Verification items for the finished model (mm, model axes). Face numbers are marked on the shaded views. Give positions to 0.01 mm unless a question says otherwise; leave off trailing zeros. Write each loop counter-clockwise with the first axis right and the second up, starting at its lowest first coordinate (ties: lowest second). Pieces come first, ordered by that corner, then holes. Notation, with made-up numbers: (29, 34.5) -> (77, 34.5) arc R17 ccw to (77, 53.5) -> close; hole circle Ø8 at (23, 55.25). An arc over 180 degrees is marked (long way). Use one line per item in the form item = value. Start each with the question number.
(1) Release check for a two-part mould opening along X. For the marked faces 1, 2 and 3 record: pulls with the +X half, pulls with the -X half, needs draft (parallel to the pull), parting line crosses it, or undercut.
(2) Scan lines: L1, parallel to Z at x = 52.5, y = 22; L2, parallel to X at y = 8.5, z = -28.25; L3, parallel to Y at x = 57, z = -19. Record each from-to range of solid material in increasing order.
(3) Section check B-B, the plane y = 15.5. Record the cut outline in (x, z).
(4) Depth check by flat-ended pin: pin 1 Ø4 at (y, z) = (20, -25) entering from -X; pin 2 Ø8 at (y, z) = (15.5, -28) entering from +X; pin 3 Ø2 at (x, z) = (41.5, -21) entering from +Y. Enter the tip coordinate at first touch or a pass-through.
(5) Section check A-A, the plane y = 2. Record the cut outline in (x, z).
from build123d import *

# Parameters (mm, degrees)
BOSS_EXTRUDE1_DEPTH             = 26
CUT_EXTRUDE1_DEPTH              = 26
CUT_EXTRUDE2_DEPTH              = 26
FILLET1_R                       = 5
M5_TAPPED_HOLE1_D               = 4.2
M5_TAPPED_HOLE1_DEPTH           = 6
M5_TAPPED_HOLE1_TIP             = 1.2618073
M5_TAPPED_HOLE1_ON_FACE_2_D     = 4.2
M5_TAPPED_HOLE1_ON_FACE_2_DEPTH = 6
M5_TAPPED_HOLE1_ON_FACE_2_TIP   = 1.2618073


with BuildPart() as part:
    # 草图1 → Boss-Extrude1 (new body)
    with BuildSketch(Plane(origin=(0, 0, 0), x_dir=(1, 0, 0), z_dir=(0, 1, 0))):
        Polygon((35.23935759, 18.286975519), (57.88435759, 18.286975519), (54.914973752, 35.127188096), (32.269973752, 35.127188096), align=None)
        Polygon((35.23935759, 18.286975519), (35.922187891, 14.414452446), (57.88435759, 18.286975519), align=None)
    extrude(amount=BOSS_EXTRUDE1_DEPTH)

    # Sketch1 → Cut-Extrude1 (cut)
    with BuildSketch(Plane(origin=(-1.381830042, 0, -7.836747596), x_dir=(0.984807753012208, 0, -0.17364817766693116), z_dir=(0.17364817766693116, 0, 0.984807753012208))):
        with BuildLine():
            Line((39.529978324, 0), (58.529978324, 0))
            ThreePointArc((58.529978324, 0), (49.029978324, 9.5), (39.529978324, 0))
        make_face()
    extrude(amount=-CUT_EXTRUDE1_DEPTH, mode=Mode.SUBTRACT)

    # Sketch2 → Cut-Extrude2 (cut)
    with BuildSketch(Plane(origin=(0, 26, 0), x_dir=(1, 0, 0), z_dir=(0, 1, 0))):
        Polygon((35.23935759, 18.286975519), (35.922187891, 14.414452446), (57.88435759, 18.286975519), align=None)
    extrude(amount=-CUT_EXTRUDE2_DEPTH, mode=Mode.SUBTRACT)

    # Fillet1
    fillet1_edges = [part.edges().sort_by_distance(p)[0] for p in [
        (43.592473752, 26, -35.127188096),
        (46.56185759, 26, -18.286975519),
    ]]
    fillet(fillet1_edges, radius=FILLET1_R)

    # M5 Tapped Hole1
    with Locations(Plane(origin=(33.670475294, 21, -27.184549163), x_dir=(-0.173648177667, 0, -0.984807753012), z_dir=(-0.984807753012, 0, 0.173648177667))):
        with Locations((0, 0)):
            Hole(M5_TAPPED_HOLE1_D / 2, depth=M5_TAPPED_HOLE1_DEPTH)
            with Locations((0, 0, -(M5_TAPPED_HOLE1_DEPTH + M5_TAPPED_HOLE1_TIP / 2))):  # 118° drill point
                Cone(0, M5_TAPPED_HOLE1_D / 2, M5_TAPPED_HOLE1_TIP, mode=Mode.SUBTRACT)

    # M5 Tapped Hole1 on face 2
    with Locations(Plane(origin=(56.507099646, 21, -26.097793462), x_dir=(0.17364796312, 0, 0.984807790843), z_dir=(0.984807790843, 0, -0.17364796312))):
        with Locations((0, 0)):
            Hole(M5_TAPPED_HOLE1_ON_FACE_2_D / 2, depth=M5_TAPPED_HOLE1_ON_FACE_2_DEPTH)
            with Locations((0, 0, -(M5_TAPPED_HOLE1_ON_FACE_2_DEPTH + M5_TAPPED_HOLE1_ON_FACE_2_TIP / 2))):  # 118° drill point
                Cone(0, M5_TAPPED_HOLE1_ON_FACE_2_D / 2, M5_TAPPED_HOLE1_ON_FACE_2_TIP, mode=Mode.SUBTRACT)


solid = part.part
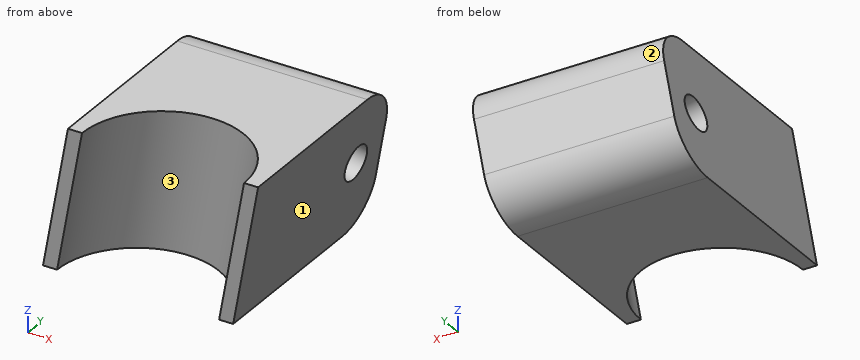
Completed:
q1.face_1 = pulls with the +X half
q1.face_2 = needs draft
q1.face_3 = undercut
q2.L1 = -35.03 to -27.27, -23.52 to -18.39
q2.L2 = 33.48 to 40.5, 49.11 to 56.13
q2.L3 = 0 to 23.57
q3.outline = (32.27, -35.13) -> (54.91, -35.13) -> (57.88, -18.29) -> (35.24, -18.29) -> close
q4.pin_1 = 33.75
q4.pin_2 = 56.88
q4.pin_3 = 25.83
q5.outline = (32.27, -35.13) -> (34.16, -35.13) -> (37.13, -18.29) -> (35.24, -18.29) -> close; (53.02, -35.13) -> (54.91, -35.13) -> (57.88, -18.29) -> (55.99, -18.29) -> close
